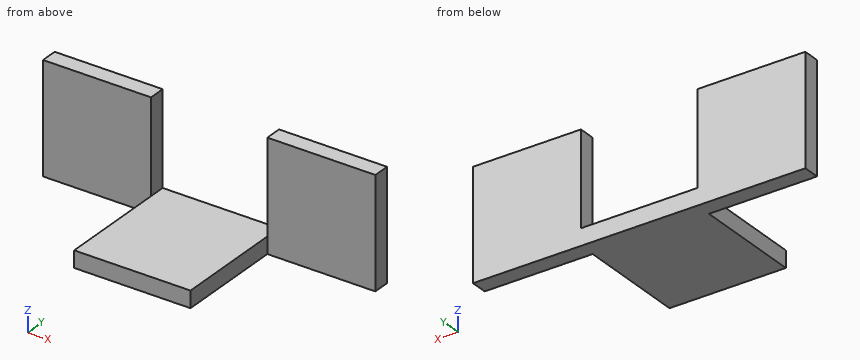
```python
from build123d import *

# Parameters (mm, degrees)
SKETCH1_W             = 24.765
SKETCH1_H             = 25.146
BOSS_EXTRUDE1_DEPTH   = 3.81
BOSS_EXTRUDE1_2_DEPTH = 3.81
SKETCH2_W             = 26.67
SKETCH2_H             = 3.81
BOSS_EXTRUDE2_DEPTH   = 28.956


with BuildPart() as part:
    # Sketch1 → Boss-Extrude1 (new body)
    with BuildSketch(Plane(origin=(0, 0, 0), x_dir=(1, 0, 0), z_dir=(0, 1, 0))):
        with Locations((12.3825, -12.573)):
            Rectangle(SKETCH1_W, SKETCH1_H)
    extrude(amount=BOSS_EXTRUDE1_DEPTH)



with BuildPart() as body_2:
    # Sketch1 → Boss-Extrude1 2 (new body)
    with BuildSketch(Plane(origin=(0, 0, 0), x_dir=(1, 0, 0), z_dir=(0, 1, 0))):
        with Locations((63.8175, -12.573)):
            Rectangle(SKETCH1_W, SKETCH1_H)
    extrude(amount=BOSS_EXTRUDE1_2_DEPTH)


with BuildPart() as part_1:
    add(part.part)

    add(body_2.part)  # Boss-Extrude2 merges body 2
    # Sketch2 → Boss-Extrude2 (add)
    with BuildSketch(Plane(origin=(0, 3.81, 0), x_dir=(1, 0, 0), z_dir=(0, 1, 0))):
        with Locations((38.1, -1.905)):
            Rectangle(SKETCH2_W, SKETCH2_H)
    extrude(amount=-BOSS_EXTRUDE2_DEPTH)


solid = part_1.part
```
Here's how the part is built. I have some questions about the finished solid (model axes, mm). Round coordinates to 2 decimals unless told otherwise and drop trailing zeros. Loops run counter-clockwise (first coordinate to the right, second up) from the corner with the lowest first, then second, coordinate; pieces in that order, holes last. Notation, with made-up numbers: (28, 1) -> (44, 1) arc R20 ccw to (44, 33) -> close; hole circle Ø1 at (-1.75, 36.5). An arc over 180 degrees is marked (long way). Answer as CSV lines item,"result".
1. If we section it at C-C on z = 1.5: Please give me the cut outline in (x, y) (3 decimals), plus the area to 3 significant figures.
Final values:
outline,"(0, 0) -> (24.765, 0) -> (24.765, -25.146) -> (51.435, -25.146) -> (51.435, 0) -> (76.2, 0) -> (76.2, 3.81) -> (0, 3.81) -> close"
area,"961 mm^2"
2. If we section it at B-B on y = 1.5: Please give me the cut outline in (x, z) (3 decimals), plus the area to 3 significant figures.
Final values:
outline,"(0, 0) -> (76.2, 0) -> (76.2, 25.146) -> (51.435, 25.146) -> (51.435, 3.81) -> (24.765, 3.81) -> (24.765, 25.146) -> (0, 25.146) -> close"
area,"1,350 mm^2"
3. If I drill on L1, parallel to Y at x = 54, z = 5; L2, parallel to X at y = -12.75, z = 2 (3 decimals), over which ranges is the centre line in solid material (lowest first)?
Final values:
L1,"y = 0 to 3.81"
L2,"x = 24.765 to 51.435"
4. For pin 1 (4 mm diameter, centred on y = -11.5, z = 1.5, fed in from +X) (3 decimals); pin 2 (1 mm diameter, centred on x = 49.5, y = -12.5, fed in from +Z); pin 3 (3 mm diameter, centred on y = -10, z = 2, fed in from -X) (3 decimals); pin 4 (12 mm diameter, centred on y = -5, z = 5, fed in from +X), each with a flat end and sliding along its axis, tell me the tip position at first contact or that it passes through.
Final values:
pin 1,"stops at x = 51.435"
pin 2,"stops at z = 3.81"
pin 3,"stops at x = 24.765"
pin 4,"stops at x = 76.2"
5. If we section it at A-A on z = 14.75: Please give me the cut outline in (x, y) (3 decimals).
Final values:
outline,"(0, 0) -> (24.765, 0) -> (24.765, 3.81) -> (0, 3.81) -> close; (51.435, 0) -> (76.2, 0) -> (76.2, 3.81) -> (51.435, 3.81) -> close"
6. If we section it at D-D on x = 54: Please give me the cut outline in (y, z).
Final values:
outline,"(0, 0) -> (3.81, 0) -> (3.81, 25.15) -> (0, 25.15) -> close"
